Here's how the part is built. I have some questions about the finished solid (model axes, mm). Face numbers are marked on the shaded views. Coordinates: 2 decimals unless noted, no trailing zeros. Loops run counter-clockwise (first coordinate to the right, second up) from the corner with the lowest first, then second, coordinate; pieces in that order, holes last. Notation, with made-up numbers: M 68.5,28.25 L 110.5,28.25 A30 cw 110.5,60.25 Z; hole C 61.5,45.25 d2. An arc over 180 degrees is marked long. Use one line per item in the form item = value. Start each with the question number.
(1) Will these pins go through, and if not, where does the flat tip stop? P1, Ø2, axis at x = -40, z = -105, coming from the -Y side; P2, Ø4, axis at x = -105, z = 40, coming from the +Y side.
(2) Imagine slicing it at B-B, the plane x = -78. State how many separate pieces and enclosed holes the cut face has, and give its area (3 significant figures).
(3) Imagine slicing it at A-A, the plane y = 6.25. Please give me the cut outline in (x, z), and give its area (3 significant figures).
(4) Thinking about a two-plate mould opening in Z: for the marked faces 1 and 2, which applies, +Z half, -Z half, draft (parallel to the pull), parting line (faces both ways), or undercut?
(5) Please list where these lines run through material, in increasing order: L1, parallel to X at y = 1.6, z = 15; L2, parallel to Z at x = -97, y = 0.5; L3, parallel to Z at x = 81, y = 3.
```python
from build123d import *

# Parameters (mm, degrees)
SKETCH_1_W               = 225
SKETCH_1_H               = 225
EXTRUDE_1_DEPTH          = 3.5
SKETCH_2_R               = 37
CUT_EXTRUDE_1_DEPTH      = 8
SKETCH_4_R               = 1.65
CUT_EXTRUDE_2_DEPTH      = 160.137519146
SKETCH_3_W               = 225
SKETCH_3_H               = 225
SKETCH_3_W_2             = 219
SKETCH_3_H_2             = 219
EXTRUDE_1975_DEPTH       = 5
SKETCH_5_R               = 1.65
CUT_EXTRUDE_2992_DEPTH   = 10
MIRROR_2_COPY_1_SKETCH_R = 37
MIRROR_2_COPY_1_DEPTH    = 8
MIRROR_2_COPY_2_SKETCH_R = 1.65
MIRROR_2_COPY_2_DEPTH    = 160.137519146
FILLET_1_R               = 5
FILLET_2_R               = 3
SKETCH_6_R               = 1.65
CUT_EXTRUDE_3_DEPTH      = 10


with BuildPart() as part:
    # 草图1 → 凸台-拉伸1 (new body)
    with BuildSketch(Plane(origin=(0, 0, 0), x_dir=(1, 0, 0), z_dir=(0, 1, 0))):
        Rectangle(SKETCH_1_W, SKETCH_1_H)
    extrude(amount=EXTRUDE_1_DEPTH)

    # 草图2 → 切除-拉伸1 (cut)
    with BuildSketch(Plane(origin=(0, 3.5, 0), x_dir=(1, 0, 0), z_dir=(0, 1, 0))):
        with Locations(Location((-72.5, -72.5, 0), (0, 0, 270))):
            Circle(SKETCH_2_R)
    cut_extrude_1 = extrude(amount=-CUT_EXTRUDE_1_DEPTH, mode=Mode.SUBTRACT)

    # 草图4 → 切除-拉伸2 (cut, through all)
    with BuildSketch(Plane.XZ):
        with Locations(Location((-40, 40, 0), (0, 0, 270))):
            Circle(SKETCH_4_R)
        with Locations(Location((-105, 40, 0), (0, 0, 270))):
            Circle(SKETCH_4_R)
        with Locations(Location((-105, 105, 0), (0, 0, 270))):
            Circle(SKETCH_4_R)
        with Locations(Location((-40, 105, 0), (0, 0, 270))):
            Circle(SKETCH_4_R)
    cut_extrude_2 = extrude(amount=-CUT_EXTRUDE_2_DEPTH, mode=Mode.SUBTRACT)

    # 草图3 → Extrude 1975 (add)
    # profile 1 of 2: a face of its own
    with BuildSketch(Plane(origin=(0, 3.5, 0), x_dir=(1, 0, 0), z_dir=(0, 1, 0))):
        Rectangle(SKETCH_3_W, SKETCH_3_H)
        Rectangle(SKETCH_3_W_2, SKETCH_3_H_2, mode=Mode.SUBTRACT)
    # profile 2 of 2: a face of its own
    with BuildSketch(Plane(origin=(0, 3.5, 0), x_dir=(1, 0, 0), z_dir=(0, 1, 0))):
        Polygon((2, 109.5), (2, 2), (109.5, 2), (109.5, -2), (2, -2), (2, -109.5), (-2, -109.5), (-2, -2), (-109.5, -2), (-109.5, 2), (-2, 2), (-2, 109.5), align=None)
    extrude(amount=EXTRUDE_1975_DEPTH)

    # 草图5 → Cut-Extrude 2992 (cut)
    with BuildSketch(Plane.XZ):
        with Locations(Location((-102.5, 17.5, 0), (0, 0, 270))):
            Circle(SKETCH_5_R)
        with Locations(Location((-102.5, -17.5, 0), (0, 0, 270))):
            Circle(SKETCH_5_R)
        with Locations(Location((-82.5, 17.5, 0), (0, 0, 270))):
            Circle(SKETCH_5_R)
        with Locations(Location((-82.5, -17.5, 0), (0, 0, 270))):
            Circle(SKETCH_5_R)
        with Locations(Location((-62.5, 17.5, 0), (0, 0, 270))):
            Circle(SKETCH_5_R)
        with Locations(Location((-62.5, -17.5, 0), (0, 0, 270))):
            Circle(SKETCH_5_R)
        with Locations(Location((-42.5, 17.5, 0), (0, 0, 270))):
            Circle(SKETCH_5_R)
        with Locations(Location((-42.5, -17.5, 0), (0, 0, 270))):
            Circle(SKETCH_5_R)
        with Locations(Location((17.5, 42.5, 0), (0, 0, 270))):
            Circle(SKETCH_5_R)
        with Locations(Location((-17.5, 42.5, 0), (0, 0, 270))):
            Circle(SKETCH_5_R)
        with Locations(Location((-17.5, 62.5, 0), (0, 0, 270))):
            Circle(SKETCH_5_R)
        with Locations(Location((17.5, 62.5, 0), (0, 0, 270))):
            Circle(SKETCH_5_R)
        with Locations(Location((17.5, 82.5, 0), (0, 0, 270))):
            Circle(SKETCH_5_R)
        with Locations(Location((-17.5, 82.5, 0), (0, 0, 270))):
            Circle(SKETCH_5_R)
        with Locations(Location((-17.5, 102.5, 0), (0, 0, 270))):
            Circle(SKETCH_5_R)
        with Locations(Location((17.5, 102.5, 0), (0, 0, 270))):
            Circle(SKETCH_5_R)
        with Locations(Location((42.5, -17.5, 0), (0, 0, 270))):
            Circle(SKETCH_5_R)
        with Locations(Location((42.5, 17.5, 0), (0, 0, 270))):
            Circle(SKETCH_5_R)
        with Locations(Location((62.5, 17.5, 0), (0, 0, 270))):
            Circle(SKETCH_5_R)
        with Locations(Location((62.5, -17.5, 0), (0, 0, 270))):
            Circle(SKETCH_5_R)
        with Locations(Location((82.5, -17.5, 0), (0, 0, 270))):
            Circle(SKETCH_5_R)
        with Locations(Location((82.5, 17.5, 0), (0, 0, 270))):
            Circle(SKETCH_5_R)
        with Locations(Location((102.5, 17.5, 0), (0, 0, 270))):
            Circle(SKETCH_5_R)
        with Locations(Location((102.5, -17.5, 0), (0, 0, 270))):
            Circle(SKETCH_5_R)
        with Locations(Location((-17.5, -42.5, 0), (0, 0, 270))):
            Circle(SKETCH_5_R)
        with Locations(Location((17.5, -42.5, 0), (0, 0, 270))):
            Circle(SKETCH_5_R)
        with Locations(Location((17.5, -62.5, 0), (0, 0, 270))):
            Circle(SKETCH_5_R)
        with Locations(Location((-17.5, -62.5, 0), (0, 0, 270))):
            Circle(SKETCH_5_R)
        with Locations(Location((-17.5, -82.5, 0), (0, 0, 270))):
            Circle(SKETCH_5_R)
        with Locations(Location((17.5, -82.5, 0), (0, 0, 270))):
            Circle(SKETCH_5_R)
        with Locations(Location((17.5, -102.5, 0), (0, 0, 270))):
            Circle(SKETCH_5_R)
        with Locations(Location((-17.5, -102.5, 0), (0, 0, 270))):
            Circle(SKETCH_5_R)
    extrude(amount=-CUT_EXTRUDE_2992_DEPTH, mode=Mode.SUBTRACT)

    # 镜向1: 切除-拉伸1, 切除-拉伸2 across plane
    add(cut_extrude_1.mirror(Plane(origin=(0, 0, 0), x_dir=(0, 0, 1), z_dir=(1, 0, 0))), mode=Mode.SUBTRACT)
    add(cut_extrude_2.mirror(Plane(origin=(0, 0, 0), x_dir=(0, 0, 1), z_dir=(1, 0, 0))), mode=Mode.SUBTRACT)

    # 镜向2: 切除-拉伸1, 切除-拉伸2 across plane
    add(cut_extrude_1.mirror(Plane.XY), mode=Mode.SUBTRACT)
    add(cut_extrude_2.mirror(Plane.XY), mode=Mode.SUBTRACT)

    # 镜向2 copy 1 sketch → 镜向2 copy 1 (cut)
    with BuildSketch(Plane(origin=(0, 3.5, 0), x_dir=(-1, 0, 0), z_dir=(0, 1, 0))):
        with Locations(Location((-72.5, -72.5, 0), (0, 0, 270))):
            Circle(MIRROR_2_COPY_1_SKETCH_R)
    extrude(amount=-MIRROR_2_COPY_1_DEPTH, mode=Mode.SUBTRACT)

    # 镜向2 copy 2 sketch → 镜向2 copy 2 (cut, through all)
    with BuildSketch(Plane(origin=(0, 0, 0), x_dir=(-1, 0, 0), z_dir=(0, -1, 0))):
        with Locations(Location((-40, 40, 0), (0, 0, 270))):
            Circle(MIRROR_2_COPY_2_SKETCH_R)
        with Locations(Location((-105, 40, 0), (0, 0, 270))):
            Circle(MIRROR_2_COPY_2_SKETCH_R)
        with Locations(Location((-105, 105, 0), (0, 0, 270))):
            Circle(MIRROR_2_COPY_2_SKETCH_R)
        with Locations(Location((-40, 105, 0), (0, 0, 270))):
            Circle(MIRROR_2_COPY_2_SKETCH_R)
    extrude(amount=-MIRROR_2_COPY_2_DEPTH, mode=Mode.SUBTRACT)

    # 圆角1
    fillet_1_edges = [part.edges().sort_by_distance(p)[0] for p in [
        (-55.75, 3.5, -2),
        (55.75, 3.5, -2),
        (55.75, 3.5, 2),
        (-55.75, 3.5, 2),
        (-2, 3.5, 55.75),
        (2, 3.5, 55.75),
        (2, 3.5, -55.75),
        (-2, 3.5, -55.75),
    ]]
    fillet(fillet_1_edges, radius=FILLET_1_R - 0.0001)  # a hair under: the kernel refuses the full size

    # 圆角2
    fillet_2_edges = [part.edges().sort_by_distance(p)[0] for p in [
        (109.5, 6, 109.5),
        (-109.5, 6, 109.5),
        (-109.5, 6, -109.5),
        (109.5, 6, -109.5),
        (112.5, 4.25, 112.5),
        (-112.5, 4.25, 112.5),
        (-112.5, 4.25, -112.5),
        (112.5, 4.25, -112.5),
    ]]
    fillet(fillet_2_edges, radius=FILLET_2_R)

    # 草图6 → 切除-拉伸3 (cut)
    with BuildSketch(Plane.XZ):
        with Locations(Location((-30, 30, 0), (0, 0, 270))):
            Circle(SKETCH_6_R)
        with Locations(Location((-15, 30, 0), (0, 0, 270))):
            Circle(SKETCH_6_R)
        with Locations(Location((15, 30, 0), (0, 0, 270))):
            Circle(SKETCH_6_R)
        with Locations(Location((30, 30, 0), (0, 0, 270))):
            Circle(SKETCH_6_R)
        with Locations(Location((-15, 15, 0), (0, 0, 270))):
            Circle(SKETCH_6_R)
        with Locations(Location((15, 15, 0), (0, 0, 270))):
            Circle(SKETCH_6_R)
        with Locations(Location((30, 15, 0), (0, 0, 270))):
            Circle(SKETCH_6_R)
        with Locations(Location((-15, -15, 0), (0, 0, 270))):
            Circle(SKETCH_6_R)
        with Locations(Location((15, -15, 0), (0, 0, 270))):
            Circle(SKETCH_6_R)
        with Locations(Location((30, -15, 0), (0, 0, 270))):
            Circle(SKETCH_6_R)
        with Locations(Location((-15, -30, 0), (0, 0, 270))):
            Circle(SKETCH_6_R)
        with Locations(Location((15, -30, 0), (0, 0, 270))):
            Circle(SKETCH_6_R)
        with Locations(Location((30, -30, 0), (0, 0, 270))):
            Circle(SKETCH_6_R)
        with Locations(Location((-30, 15, 0), (0, 0, 270))):
            Circle(SKETCH_6_R)
        with Locations(Location((-30, -15, 0), (0, 0, 270))):
            Circle(SKETCH_6_R)
        with Locations(Location((-30, -30, 0), (0, 0, 270))):
            Circle(SKETCH_6_R)
    extrude(amount=-CUT_EXTRUDE_3_DEPTH, mode=Mode.SUBTRACT)


solid = part.part
```
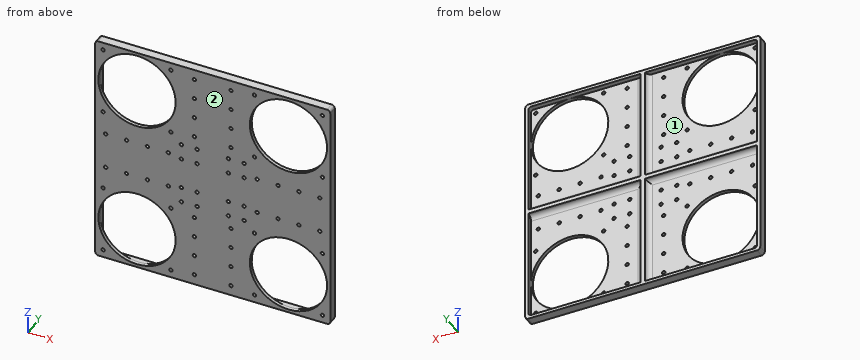
Answer:
q1.P1 = through
q1.P2 = 3.5
q2.separate_pieces = 3
q2.enclosed_holes = 0
q2.area = 336 mm²
q3.outline = M -112.5,-109.5 A3 ccw -109.5,-112.5 L 109.5,-112.5 A3 ccw 112.5,-109.5 L 112.5,109.5 A3 ccw 109.5,112.5 L -109.5,112.5 A3 ccw -112.5,109.5 Z; hole M -109.5,-106.5 A3 ccw -106.5,-109.5 L -2.53,-109.5 L -2.53,-2.53 L -109.5,-2.53 Z; hole M -109.5,2.53 L -2.53,2.53 L -2.53,109.5 L -106.5,109.5 A3 ccw -109.5,106.5 Z; hole M 2.53,-109.5 L 106.5,-109.5 A3 ccw 109.5,-106.5 L 109.5,-2.53 L 2.53,-2.53 Z; hole M 2.53,2.53 L 109.5,2.53 L 109.5,106.5 A3 ccw 106.5,109.5 L 2.53,109.5 Z
q3.area = 4,860 mm²
q4.face_1 = undercut
q4.face_2 = draft
q5.L1 = -112.5 to -31.65, -28.35 to -16.65, -13.35 to 13.35, 16.65 to 28.35, 31.65 to 112.5
q5.L2 = -112.5 to -100.23, -44.77 to 44.77, 100.23 to 112.5
q5.L3 = -112.5 to -108.51, -36.49 to -18.19, -16.81 to 16.81, 18.19 to 36.49, 108.51 to 112.5
